from build123d import *

# Parameters (mm, degrees)
ESQUISSE1_W                  = 60
ESQUISSE1_H                  = 6
BOSS_EXTRU_1_DEPTH           = 40
ENL_V_MAT_EXTRU_1_DEPTH      = 73.360210061
ENL_V_MAT_EXTRU_1_DEPTH_BACK = 73.360210061
ESQUISSE2_R                  = 5
ENL_V_MAT_EXTRU_3_DEPTH      = 73.360210061
ENL_V_MAT_EXTRU_3_DEPTH_BACK = 73.360210061
ESQUISSE4_R                  = 1.75
ESQUISSE7_W                  = 60
ESQUISSE7_H                  = 4
BOSS_EXTRU_2_DEPTH           = 50
BOSS_EXTRU_3_DEPTH           = 3
BOSS_EXTRU_4_START           = -60
BOSS_EXTRU_4_DEPTH           = 3
ENL_V_MAT_EXTRU_4_DEPTH      = 88.749643874
ENL_V_MAT_EXTRU_4_DEPTH_BACK = 88.749643874
ESQUISSE9_R                  = 2
CHANFREIN1_SIZE              = 1


with BuildPart() as part:
    # Esquisse1 → Boss.-Extru.1 (new body)
    with BuildSketch(Plane.XY):
        with Locations((30, 3)):
            Rectangle(ESQUISSE1_W, ESQUISSE1_H)
    extrude(amount=BOSS_EXTRU_1_DEPTH)

    # Esquisse2 → Enlèv. mat.-Extru.1 (cut, two sides: drawn at the far end of the back side and taken through both)
    with BuildSketch(Plane(origin=(0, 6, 0), x_dir=(1, 0, 0), z_dir=(0, 1, 0)).offset(-ENL_V_MAT_EXTRU_1_DEPTH_BACK)):
        with Locations(Location((30, -20, 0), (0, 0, 270))):
            Circle(ESQUISSE2_R)
    extrude(amount=ENL_V_MAT_EXTRU_1_DEPTH + ENL_V_MAT_EXTRU_1_DEPTH_BACK, mode=Mode.SUBTRACT)

    # Esquisse4 → Enlèv. mat.-Extru.3 (cut, two sides: drawn at the far end of the back side and taken through both)
    with BuildSketch(Plane(origin=(0, 6, 0), x_dir=(1, 0, 0), z_dir=(0, 1, 0)).offset(-ENL_V_MAT_EXTRU_3_DEPTH_BACK)):
        with Locations(Location((45, -20, 0), (0, 0, 270))):
            Circle(ESQUISSE4_R)
        with Locations(Location((22.5, -32.990381057, 0), (0, 0, 270))):
            Circle(ESQUISSE4_R)
        with Locations(Location((22.5, -7.009618943, 0), (0, 0, 270))):
            Circle(ESQUISSE4_R)
    extrude(amount=ENL_V_MAT_EXTRU_3_DEPTH + ENL_V_MAT_EXTRU_3_DEPTH_BACK, mode=Mode.SUBTRACT)

    # Esquisse7 → Boss.-Extru.2 (add)
    with BuildSketch(Plane.XZ):
        with Locations((30, 42)):
            Rectangle(ESQUISSE7_W, ESQUISSE7_H)
    extrude(amount=-BOSS_EXTRU_2_DEPTH)

    # Esquisse8 → Boss.-Extru.3 (add)
    with BuildSketch(Plane(origin=(60, 0, 0), x_dir=(0, 0, -1), z_dir=(1, 0, 0))):
        Polygon((0, 6), (-40, 50), (-40, 6), align=None)
    extrude(amount=-BOSS_EXTRU_3_DEPTH)

    # Esquisse8<2> → Boss.-Extru.4 (add)
    with BuildSketch(Plane(origin=(60, 0, 0), x_dir=(0, 0, -1), z_dir=(1, 0, 0)).offset(BOSS_EXTRU_4_START)):
        Polygon((0, 6), (-40, 50), (-40, 6), align=None)
    extrude(amount=BOSS_EXTRU_4_DEPTH)

    # Esquisse9 → Enlèv. mat.-Extru.4 (cut, two sides: drawn at the far end of the back side and taken through both)
    with BuildSketch(Plane(origin=(0, 0, 40), x_dir=(-1, 0, 0), z_dir=(0, 0, -1)).offset(-ENL_V_MAT_EXTRU_4_DEPTH_BACK)):
        with Locations((-51, 12)):
            Circle(ESQUISSE9_R)
        with Locations((-51, 44)):
            Circle(ESQUISSE9_R)
        with Locations((-9, 44)):
            Circle(ESQUISSE9_R)
        with Locations((-9, 12)):
            Circle(ESQUISSE9_R)
    extrude(amount=ENL_V_MAT_EXTRU_4_DEPTH + ENL_V_MAT_EXTRU_4_DEPTH_BACK, mode=Mode.SUBTRACT)

    # Chanfrein1
    chanfrein1_edges = [part.edges().sort_by_distance(p)[0] for p in [
        (11, 12, 40),
        (11, 44, 40),
        (53, 44, 40),
        (53, 12, 40),
    ]]
    chamfer(chanfrein1_edges, length=CHANFREIN1_SIZE)


solid = part.part
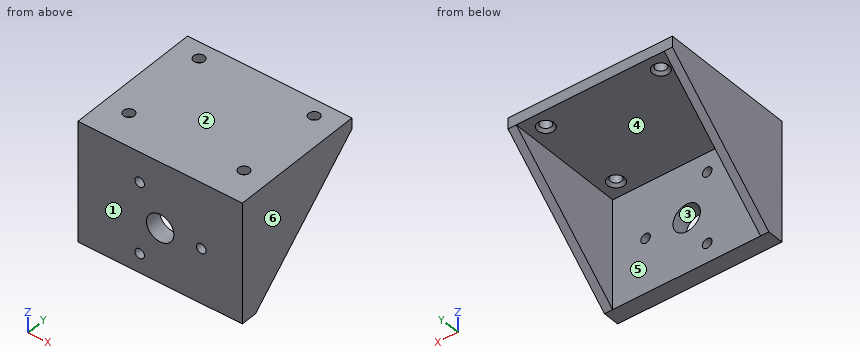
CAD build for the part. Positions are in the model's coordinates, mm. Face numbers are marked on the shaded views. A direction names the side the tool comes from. Give positions to 0.01 mm unless a question says otherwise; leave off trailing zeros. Order: outer loops, then holes, each group sorted by start corner. A loop starts at its lowest first (then second) coordinate and runs counter-clockwise, first axis right, second up. Notation, with made-up numbers: (49.5, -28.75) - (67.5, -28.75) arc R13 ccw to (67.5, -10.75) - close; hole circle Ø3 at (69, -18). An arc over 180 degrees is marked (long way). Answer in a Markdown table with one row per item.
1. Saw through at B-B, the plane z = 16. Give the cut face in (x, y), plus the area to 3 significant figures.
Data:
| item | result |
|---|---|
| outline | (0, 0) - (27, 0) - (27, 6) - (3, 6) - (3, 23.6) - (0, 23.6) - close; (33, 0) - (60, 0) - (60, 23.6) - (57, 23.6) - (57, 6) - (33, 6) - close |
| area | 430 mm² |
2. Pull direction Z, two halves, no side cores. Call the marked faces 1, 2, 3 and 4: pulls with the +Z half, pulls with the -Z half, needs draft (parallel to the pull), parting line crosses it, or undercut.
Data:
| item | result |
|---|---|
| face 1 | needs draft |
| face 2 | pulls with the +Z half |
| face 3 | undercut |
| face 4 | pulls with the -Z half |
3. Probe probe 1 along X at (y, z) = (12, 41.9); probe 2 along X at (y, z) = (3.85, 20); probe 3 along Z at (x, y) = (22.5, 3.85). List the from-to ranges inside material, lowest first. Write a range as [from, to].
Data:
| item | result |
|---|---|
| probe 1 | x = [0, 7], [11, 49], [53, 60] |
| probe 2 | x = [0, 25], [35, 43.25], [46.75, 60] |
| probe 3 | z = [0, 5.26], [8.76, 31.24], [34.74, 44] |
4. Saw through at A-A, the plane x = 51. Give the cut face in (y, z).
Data:
| item | result |
|---|---|
| outline | (0, 0) - (6, 0) - (6, 40) - (9, 40) - (10, 41) - (10, 44) - (0, 44) - close; (14, 41) - (15, 40) - (41, 40) - (42, 41) - (42, 44) - (14, 44) - close; (46, 41) - (47, 40) - (50, 40) - (50, 44) - (46, 44) - close |
5. Flat gauge pins, fed straight in: pin 1 (12 mm diameter, centred on x = 29, z = 26, fed in from +Y); pin 2 (2.5 mm diameter, centred on x = 9, y = 44, fed in from -Z); pin 3 (22 mm diameter, centred on x = 32.5, y = 38, fed in from -Z). Where does each tip first touch, or does it go through?
Data:
| item | result |
|---|---|
| pin 1 | stops at y = 6 |
| pin 2 | passes through |
| pin 3 | stops at z = 40 |
6. Saw through at D-D, the plane x = 30. Give the cut face in (y, z).
Data:
| item | result |
|---|---|
| outline | (0, 0) - (6, 0) - (6, 15) - (0, 15) - close; (0, 25) - (6, 25) - (6, 40) - (50, 40) - (50, 44) - (0, 44) - close |
7. Saw through at C-C, the plane y = 4.5. Give the cut face in (x, z).
Data:
| item | result |
|---|---|
| outline | (0, 0) - (60, 0) - (60, 44) - (0, 44) - close; hole circle Ø3.5 at (22.5, 7.01); hole circle Ø3.5 at (22.5, 32.99); hole circle Ø10 at (30, 20); hole circle Ø3.5 at (45, 20) |
8. Tool access for the marked faces 5 and 6: list every direction of +Z, -Z, +X, -X, +Y, -Y with a clear straight run to the whole face (end or side of a thin tool).
Data:
| item | result |
|---|---|
| face 5 | -Z, +Y |
| face 6 | +Z, -Z, +X, +Y, -Y |
